Work out the finished part from the listing and answer in its coordinate system (mm). Face numbers are marked on the shaded views. A direction names the side the tool comes from. Coordinates: 2 decimals unless noted, no trailing zeros. Order: outer loops, then holes, each group sorted by start corner. A loop starts at its lowest first (then second) coordinate and runs counter-clockwise, first axis right, second up. Notation, with made-up numbers: (74, 68.25) -> (90, 68.25) arc R11 cw to (90, 73.25) -> close; hole circle Ø4 at (66, 79). An arc over 180 degrees is marked (long way). Write item = value, one per line. Start each with the question number.
Q1. The part is cut by section B-B, the plane y = 7.5. Determine the outline of the cut face in (x, z), plus the area to 3 significant figures.
Q2. Which of the six approach directions +Z, -Z, +X, -X, +Y, -Y give full straight-line access (tool end or side, diameter ignored) to the marked faces 1, 2 and 3?
Q3. The part is cut by section D-D, the plane z = -30. Determine the outline of the cut face in (x, y).
Q4. Flat-ended cylindrical pins translate along their axes: pin 1 (8 mm diameter, centred on x = 81, y = 29, fed in from -Z); pin 2 (3.5 mm diameter, centred on x = 103.5, y = 29.5, fed in from -Z); pin 3 (22 mm diameter, centred on x = 31.5, z = -51, fed in from +Y); pin 4 (2.5 mm diameter, centred on x = 13, y = 29.05, fed in from -Z). Find the tip coordinate at first contact, or state that the pin passes through.
Q5. The part is cut by section A-A, the plane x = 103. Count the separate pieces of the cut face and the enclosed holes in it, plus the area to 3 significant figures.
Q6. Straight lines are drawn through the part: L1, parallel to X at y = 29, z = -6; L2, parallel to Y at x = 13, z = -7.2; L3, parallel to Y at x = 103, z = -2. For each, find the intervals that lie inside material, in ascending order. Write a range as from..to.
```python
from build123d import *

# Parameters (mm, degrees)
SKETCH1_W           = 116
SKETCH1_H           = 70
BOSS_EXTRUDE1_DEPTH = 10
SKETCH2_W           = 116
SKETCH2_H           = 9.05
BOSS_EXTRUDE2_DEPTH = 10
CUT_EXTRUDE1_DEPTH  = 136.852861582
SKETCH4_W           = 116
SKETCH4_H           = 17
BOSS_EXTRUDE3_DEPTH = 10
FILLET1_R           = 16
BOSS_EXTRUDE4_START = -85
BOSS_EXTRUDE4_DEPTH = 50
SKETCH7_W           = 4
SKETCH7_H           = 16
BOSS_EXTRUDE5_DEPTH = 116
CHAMFER1_SIZE2      = 4
CHAMFER1_SIZE       = 10
FILLET3_R           = 1
FILLET4_R           = 5
SKETCH8_R           = 1.65
CUT_EXTRUDE2_DEPTH  = 143.237837793
SKETCH9_R           = 2.25
CUT_EXTRUDE3_DEPTH  = 5


with BuildPart() as part:
    # Sketch1 → Boss-Extrude1 (new body)
    with BuildSketch(Plane(origin=(0, 0, 0), x_dir=(1, 0, 0), z_dir=(0, 1, 0))):
        with Locations((58, 35)):
            Rectangle(SKETCH1_W, SKETCH1_H)
    extrude(amount=BOSS_EXTRUDE1_DEPTH)

    # Sketch2 → Boss-Extrude2 (add)
    with BuildSketch(Plane.XY):
        with Locations((58, 14.525)):
            Rectangle(SKETCH2_W, SKETCH2_H)
    extrude(amount=-BOSS_EXTRUDE2_DEPTH)

    # Sketch3 → Cut-Extrude1 (cut, through all)
    with BuildSketch(Plane(origin=(0, 10, 0), x_dir=(1, 0, 0), z_dir=(0, 1, 0))):
        with BuildLine():
            Line((16, 59), (16, 41))
            ThreePointArc((16, 41), (13, 38), (10, 41))
            Line((10, 41), (10, 59))
            ThreePointArc((10, 59), (13, 62), (16, 59))
        make_face()
        with BuildLine():
            Line((100, 59), (100, 41))
            ThreePointArc((100, 41), (103, 38), (106, 41))
            Line((106, 41), (106, 59))
            ThreePointArc((106, 59), (103, 62), (100, 59))
        make_face()
    extrude(amount=-CUT_EXTRUDE1_DEPTH, mode=Mode.SUBTRACT)

    # Sketch4 → Boss-Extrude3 (add)
    with BuildSketch(Plane.XY):
        with Locations((58, 27.55)):
            Rectangle(SKETCH4_W, SKETCH4_H)
    extrude(amount=-BOSS_EXTRUDE3_DEPTH)

    # Fillet1
    fillet1_edges = [part.edges().sort_by_distance(p)[0] for p in [
        (58, 10, -10),
    ]]
    fillet(fillet1_edges, radius=FILLET1_R)

    # Sketch6 → Boss-Extrude4 (add)
    with BuildSketch(Plane.ZY.offset(BOSS_EXTRUDE4_START)):
        with BuildLine():
            Line((-10, 36.05), (-60, 10))
            Line((-60, 10), (-26, 10))
            ThreePointArc((-26, 10), (-14.686291501, 14.686291501), (-10, 26))
            Line((-10, 26), (-10, 36.05))
        make_face()
    extrude(amount=BOSS_EXTRUDE4_DEPTH)

    # Sketch7 → Boss-Extrude5 (add)
    with BuildSketch(Plane.ZY):
        with Locations((2, 28.05)):
            Rectangle(SKETCH7_W, SKETCH7_H)
    extrude(amount=-BOSS_EXTRUDE5_DEPTH)

    # Chamfer1
    chamfer1_edges = [part.edges().sort_by_distance(p)[0] for p in [
        (58, 20.05, 0),
    ]]
    chamfer1_side = [part.faces().sort_by_distance(p)[0] for p in [
        (58, 19.97, 0),
    ]]
    chamfer(chamfer1_edges, length=CHAMFER1_SIZE - 0.0001, length2=CHAMFER1_SIZE2 - 0.0001, reference=chamfer1_side[0])  # a hair under: the kernel refuses the full size

    # Fillet3
    fillet3_edges = [part.edges().sort_by_distance(p)[0] for p in [
        (58, 36.05, 4),
    ]]
    fillet(fillet3_edges, radius=FILLET3_R)

    # Fillet4
    fillet4_edges = [part.edges().sort_by_distance(p)[0] for p in [
        (0, 5, -70),
        (116, 5, -70),
    ]]
    fillet(fillet4_edges, radius=FILLET4_R)

    # Sketch8 → Cut-Extrude2 (cut, through all)
    with BuildSketch(Plane.XY.offset(4)):
        with Locations((13, 29.05)):
            Circle(SKETCH8_R)
        with Locations((103, 29.05)):
            Circle(SKETCH8_R)
    extrude(amount=-CUT_EXTRUDE2_DEPTH, mode=Mode.SUBTRACT)

    # Sketch9 → Cut-Extrude3 (cut)
    with BuildSketch(Plane(origin=(0, 0, -10), x_dir=(-1, 0, 0), z_dir=(0, 0, -1))):
        with Locations((-103, 29.05)):
            Circle(SKETCH9_R)
        with Locations((-13, 29.05)):
            Circle(SKETCH9_R)
    extrude(amount=-CUT_EXTRUDE3_DEPTH, mode=Mode.SUBTRACT)


solid = part.part
```
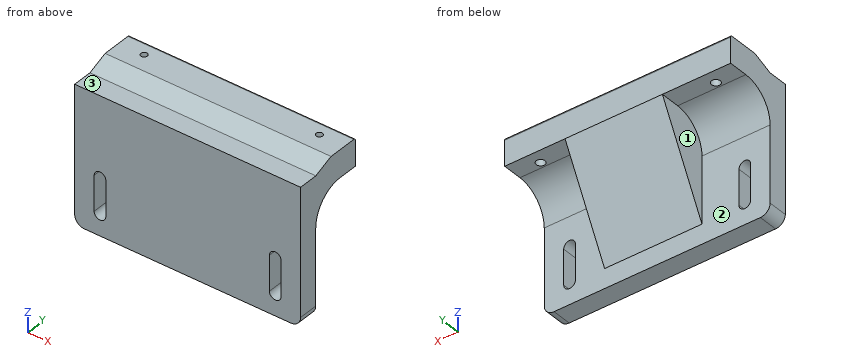
Model answer:
q1.outline = (0, -65) arc R5 ccw to (5, -70) -> (111, -70) arc R5 ccw to (116, -65) -> (116, 0) -> (0, 0) -> close; hole (10, -59) arc R3 ccw to (16, -59) -> (16, -41) arc R3 ccw to (10, -41) -> close; hole (100, -59) arc R3 ccw to (106, -59) -> (106, -41) arc R3 ccw to (100, -41) -> close
q1.area = 7,840 mm2
q2.face_1 = -Z, -X, +Y
q2.face_2 = -Z, +Y
q2.face_3 = +Z, +X, -X, -Y
q3.outline = (0, 0) -> (116, 0) -> (116, 10) -> (85, 10) -> (85, 25.63) -> (35, 25.63) -> (35, 10) -> (0, 10) -> close
q4.pin_1 = -31.21
q4.pin_2 = -10
q4.pin_3 = 20.12
q4.pin_4 = through
q5.separate_pieces = 3
q5.enclosed_holes = 0
q5.area = 807 mm2
q6.L1 = 0..10.75, 15.25..100.75, 105.25..116
q6.L2 = 0..26.8, 31.3..36.05
q6.L3 = 0..27.4, 30.7..36.05
